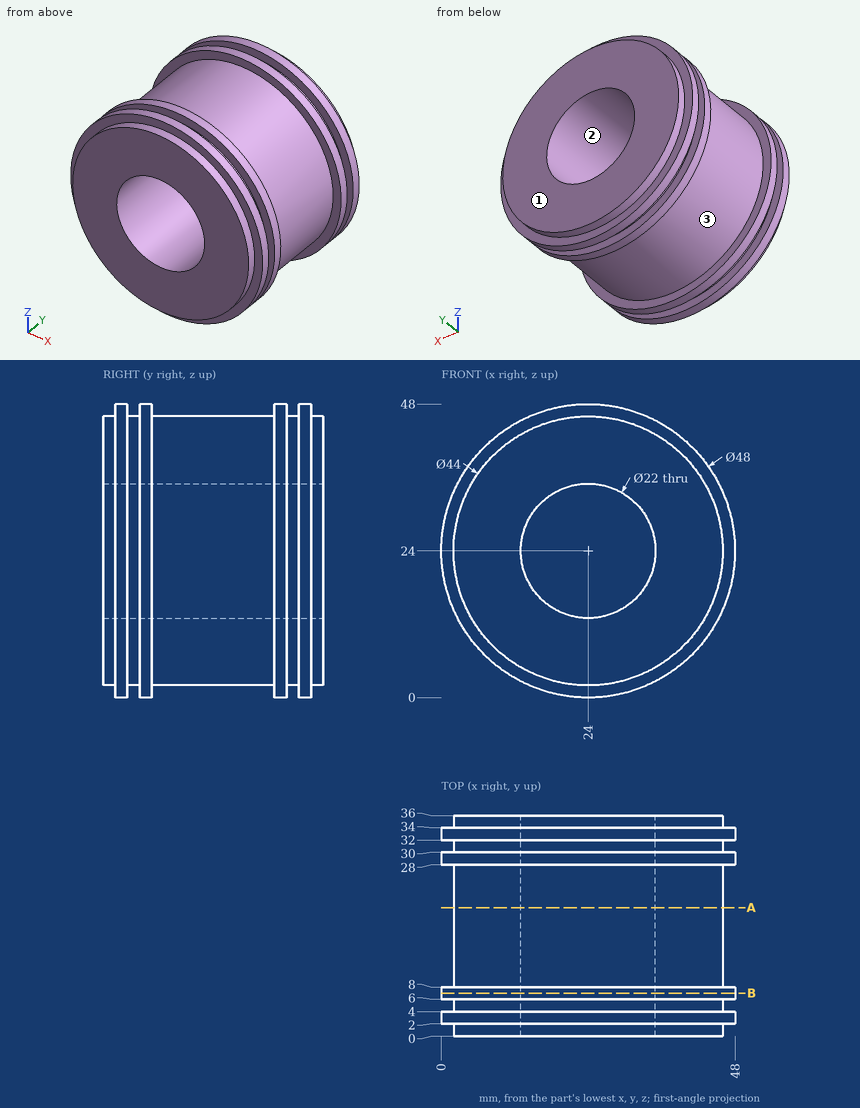
Verification items for this drawing (mm, ordinates from the low corner). Give positions to 0.01 mm unless a question says otherwise; leave off trailing zeros. Write each loop counter-clockwise with the first axis right and the second up, starting at its lowest first coordinate (ties: lowest second). Pieces come first, ordered by that corner, then holes. Notation, with made-up numbers: (76.5, -5) - (85.5, -5) arc R22 ccw to (85.5, 34) - close; hole circle Ø6 at (30, 35.25). An arc over 180 degrees is marked (long way). Answer as CSV lines item,"result". Start each with the question number.
1. Depth check by flat-ended pin: pin 1 (17.5 mm diameter, centred on x = 24, z = 24, fed in from +Y); pin 2 (12 mm diameter, centred on x = 42.5, y = 8.5, fed in from +Z); pin 3 (8 mm diameter, centred on x = 30, y = 23.5, fed in from -Z); pin 4 (3 mm diameter, centred on y = 31.5, z = 21.5, fed in from +X). Enter the tip coordinate at first touch or a pass-through.
2. Thickness scan on line 1 (Y direction, x = 39, z = 7.5); line 2 (X direction, y = 26, z = 24); line 3 (Z direction, x = 19.5, y = 6.5). Record the ranges inside material, lowest first.
3. Draft check along Z on the marked faces 1, 2 and 3. Enter one of: pulls with the +Z half, pulls with the -Z half, needs draft (parallel to the pull), parting line crosses it, or undercut.
4. Sectioned sample at B-B (y = 7). Record the boundary of the cut face in (x, z), then the cut area to 3 significant figures.
5. Sectioned sample at A-A (y = 21). Record the boundary of the cut face in (x, z), then the cut area to 3 significant figures.
Derived:
1,pin 1,"through"
1,pin 2,"z = 44.48"
1,pin 3,"z = 2.09"
1,pin 4,"x = 47.98"
2,line 1,"2 to 4, 6 to 8, 28 to 30, 32 to 34"
2,line 2,"2 to 13, 35 to 46"
2,line 3,"0.43 to 13.96, 34.04 to 47.57"
3,face 1,"needs draft"
3,face 2,"undercut"
3,face 3,"parting line crosses it"
4,outline,"circle Ø48 at (24, 24); hole circle Ø22 at (24, 24)"
4,area,"1,430 mm²"
5,outline,"circle Ø44 at (24, 24); hole circle Ø22 at (24, 24)"
5,area,"1,140 mm²"
